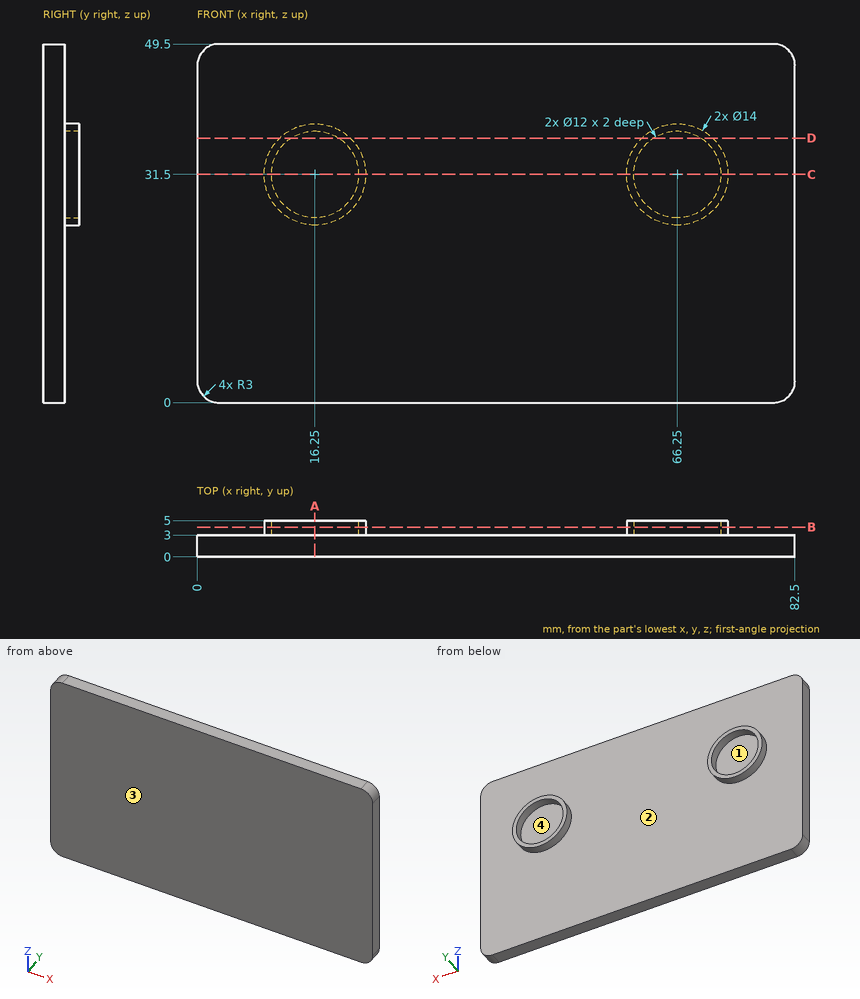
Could you check a few things on this drawing? It's one solid part, dimensions in mm from its lowest x, y, z. A direction names the side the tool comes from. Coordinates: 2 decimals unless noted, no trailing zeros. Write each loop counter-clockwise with the first axis right and the second up, starting at its lowest first coordinate (ties: lowest second). Pieces come first, ordered by that corner, then holes. Notation, with made-up numbers: (4, 69) - (21, 69) arc R32 ccw to (21, 98) - close; hole circle Ø6 at (-26.5, 52.5). An arc over 180 degrees is marked (long way). Use one line per item in the form item = value.
1) Suppose I cut it at D-D, the plane z = 36.5. Write out the boundary of the cut face in (x, y).
Solved:
outline = (0, 0) - (82.5, 0) - (82.5, 3) - (71.15, 3) - (71.15, 5) - (69.57, 5) - (69.57, 3) - (62.93, 3) - (62.93, 5) - (61.35, 5) - (61.35, 3) - (21.15, 3) - (21.15, 5) - (19.57, 5) - (19.57, 3) - (12.93, 3) - (12.93, 5) - (11.35, 5) - (11.35, 3) - (0, 3) - close
2) Suppose I cut it at B-B, the plane y = 4.1. Write out the boundary of the cut face in (x, z), plus the area to 3 significant figures.
Solved:
outline = circle Ø14 at (16.25, 31.5); circle Ø14 at (66.25, 31.5); hole circle Ø12 at (16.25, 31.5); hole circle Ø12 at (66.25, 31.5)
area = 81.7 mm2
3) Suppose I cut it at A-A, the plane x = 16.25. Write out the boundary of the cut face in (y, z), plus the area to 4 significant figures.
Solved:
outline = (0, 0) - (3, 0) - (3, 24.5) - (5, 24.5) - (5, 25.5) - (3, 25.5) - (3, 37.5) - (5, 37.5) - (5, 38.5) - (3, 38.5) - (3, 49.5) - (0, 49.5) - close
area = 152.5 mm2
4) I'm going to push a flat-ended pin straight in: P1, Ø2, axis at x = 44.5, z = 35.5, coming from the +Y side. Where does the tip first touch, or does it pass through?
Solved:
P1 = 3
5) On a 3-axis mill with a long thin cutter (end or side, diameter ignored), from which of +Z, -Z, +X, -X, +Y, -Y can I reach the whole of each face in a straight line? I mean the marked faces 3 and 4. Say none if no direction works.
Solved:
face_3 = +Z, -Z, +X, -X, -Y
face_4 = +Y
6) Suppose I cut it at C-C, the plane z = 31.5. Write out the boundary of the cut face in (x, y).
Solved:
outline = (0, 0) - (82.5, 0) - (82.5, 3) - (73.25, 3) - (73.25, 5) - (72.25, 5) - (72.25, 3) - (60.25, 3) - (60.25, 5) - (59.25, 5) - (59.25, 3) - (23.25, 3) - (23.25, 5) - (22.25, 5) - (22.25, 3) - (10.25, 3) - (10.25, 5) - (9.25, 5) - (9.25, 3) - (0, 3) - close
7) I need wall thicknesses on line 1 (X direction, y = 3.7, z = 31.5); line 2 (Z direction, x = 66.25, y = 3.9); line 3 (X direction, y = 3.6, z = 33). Which ranges of each line are inside material? Lowest first, please.
Solved:
line_1 = 9.25 to 10.25, 22.25 to 23.25, 59.25 to 60.25, 72.25 to 73.25
line_2 = 24.5 to 25.5, 37.5 to 38.5
line_3 = 9.41 to 10.44, 22.06 to 23.09, 59.41 to 60.44, 72.06 to 73.09
8) Thinking about a two-plate mould opening in Z: for the marked faces 1 and 2, which applies, released by +Z, released by -Z, zero draft, split by the parting line, or undercut?
Solved:
face_1 = undercut
face_2 = zero draft
